from build123d import *

# Parameters (mm, degrees)
SKETCH1_W           = 100
SKETCH1_H           = 100
SKETCH1_W_2         = 96
SKETCH1_H_2         = 96
BOSS_EXTRUDE1_DEPTH = 59
SKETCH2_W           = 120
SKETCH2_H           = 120
SKETCH2_W_2         = 100
SKETCH2_H_2         = 100
BOSS_EXTRUDE4_DEPTH = 1
FILLET1_R           = 4
FILLET2_R           = 6


with BuildPart() as part:
    # Sketch1 → Boss-Extrude1 (new body)
    with BuildSketch(Plane.XY):
        Rectangle(SKETCH1_W, SKETCH1_H)
        Rectangle(SKETCH1_W_2, SKETCH1_H_2, mode=Mode.SUBTRACT)
    extrude(amount=-BOSS_EXTRUDE1_DEPTH)

    # Sketch2 → Boss-Extrude4 (add)
    with BuildSketch(Plane.XY):
        Rectangle(SKETCH2_W, SKETCH2_H)
        Rectangle(SKETCH2_W_2, SKETCH2_H_2, mode=Mode.SUBTRACT)
    extrude(amount=-BOSS_EXTRUDE4_DEPTH)

    # Fillet1
    fillet1_edges = [part.edges().sort_by_distance(p)[0] for p in [
        (-50, -50, -30),
        (-50, 50, -30),
        (50, 50, -30),
        (50, -50, -30),
    ]]
    fillet(fillet1_edges, radius=FILLET1_R)

    # Fillet2
    fillet2_edges = [part.edges().sort_by_distance(p)[0] for p in [
        (60, -60, -0.5),
        (-60, -60, -0.5),
        (-60, 60, -0.5),
        (60, 60, -0.5),
    ]]
    fillet(fillet2_edges, radius=FILLET2_R)


solid = part.part
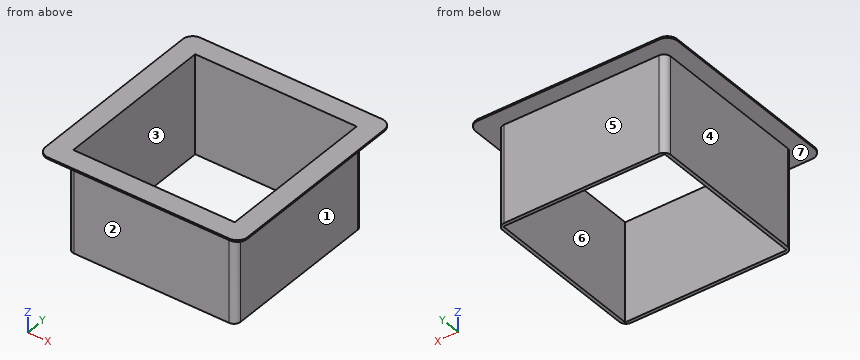
Geometry: final body of the model. Coordinates: model frame, mm. Face numbers are marked on the shaded views. A direction names the side the tool comes from. Round coordinates to 2 decimals unless told otherwise and drop trailing zeros. Loops run counter-clockwise (first coordinate to the right, second up) from the corner with the lowest first, then second, coordinate; pieces in that order, holes last.
Q1. Pin query (flat end, axial travel): P1, Ø17.5, axis at y = 5.5, z = -35.5, coming from the +X side; P2, Ø6, axis at x = 26, z = -14, coming from the -Y side; P3, Ø1.5, axis at y = -5.5, z = -48, coming from the -X side. Return the tip coordinate at first contact, or that it passes through.
Q2. Pull-direction query (X, two-part tool) for the marked faces 1, 2, 3 and 4; classes: released by +X, released by -X, zero draft, split by the parting line, or undercut.
Q3. Section C-C on z = -17.5. Return loops of the section in (x, y), plus the area to 3 significant figures.
Q4. Material intervals for L1, parallel to Y at x = -16, z = -51; L2, parallel to Z at x = 21, y = 50.5, sorted ascending.
Q5. Access query for the marked faces 5, 6 and 7. Directions: +Z, -Z, +X, -X, +Y, -Y. A direction counts if a zero-diameter tool reaches every point of the face in a straight line with its end or side. Return the directions, or none.
Q6. Section A-A on y = -33. Return loops of the section in (x, z).
Evaluation:
1. P1: stops at x = 50
1. P2: stops at y = -50
1. P3: stops at x = -50
2. face 1: released by +X
2. face 2: zero draft
2. face 3: undercut
2. face 4: released by -X
3. outline: (-50, -46) arc R4 ccw to (-46, -50) - (46, -50) arc R4 ccw to (50, -46) - (50, 46) arc R4 ccw to (46, 50) - (-46, 50) arc R4 ccw to (-50, 46) - close; hole (-48, -48) - (48, -48) - (48, 48) - (-48, 48) - close
3. area: 770 mm2
4. L1: y = -50 to -48, 48 to 50
4. L2: z = -1 to 0
5. face 5: -Z, +X, -X, +Y
5. face 6: +Z, -Z
5. face 7: -Z
6. outline: (-60, -1) - (-50, -1) - (-50, -59) - (-48, -59) - (-48, 0) - (-60, 0) - close; (48, -59) - (50, -59) - (50, -1) - (60, -1) - (60, 0) - (48, 0) - close
